Part model, mm, in its own coordinate system. Face numbers are marked on the shaded views. A direction names the side the tool comes from. Give positions to 0.01 mm unless a question says otherwise; leave off trailing zeros. Order: outer loops, then holes, each group sorted by start corner. A loop starts at its lowest first (then second) coordinate and runs counter-clockwise, first axis right, second up. Notation, with made-up numbers: M 66.25,75 L 81.25,75 A21 ccw 81.25,103 Z; hole C -36.5,29 d3. An arc over 180 degrees is marked long. One line per question, with ' | ' between items.
```python
from build123d import *

# Parameters (mm, degrees)
SKETCH1_W           = 200
SKETCH1_H           = 150
BOSS_EXTRUDE1_DEPTH = 150
SKETCH2_R           = 15
SKETCH2_R_2         = 13
BOSS_EXTRUDE2_DEPTH = 5
SKETCH3_R           = 13
SKETCH3_R_2         = 5
CUT_EXTRUDE1_DEPTH  = 70
CUT_EXTRUDE2_DEPTH  = 201
SKETCH5_R           = 15
SKETCH5_R_2         = 14
BOSS_EXTRUDE3_DEPTH = 10
SKETCH7_R           = 10
SKETCH7_R_2         = 9
SKETCH7_R_3         = 16
SKETCH7_R_4         = 15
BOSS_EXTRUDE4_DEPTH = 20
SKETCH10_W          = 70
SKETCH10_H          = 50
CUT_EXTRUDE5_DEPTH  = 151


with BuildPart() as part:
    # Sketch1 → Boss-Extrude1 (new body)
    with BuildSketch(Plane(origin=(0, 0, 0), x_dir=(1, 0, 0), z_dir=(0, 1, 0))):
        Rectangle(SKETCH1_W, SKETCH1_H)
    extrude(amount=BOSS_EXTRUDE1_DEPTH)

    # Sketch2 → Boss-Extrude2 (add)
    with BuildSketch(Plane(origin=(100, 0, 0), x_dir=(0, 0, -1), z_dir=(1, 0, 0))):
        with Locations((-10, 20)):
            Circle(SKETCH2_R)
        with Locations((-10, 20)):
            Circle(SKETCH2_R_2, mode=Mode.SUBTRACT)
    extrude(amount=BOSS_EXTRUDE2_DEPTH)

    # Sketch3 → Cut-Extrude1 (cut)
    with BuildSketch(Plane(origin=(100, 0, 0), x_dir=(0, 0, -1), z_dir=(1, 0, 0))):
        with Locations((-10, 20)):
            Circle(SKETCH3_R)
        with Locations((-37.5, 20)):
            Circle(SKETCH3_R_2)
        with Locations((17.5, 20)):
            Circle(SKETCH3_R_2)
        Polygon((75, 10), (20, 10), (20, 0), (20, -30), (75, -30), (75, 0), align=None)
    extrude(amount=-CUT_EXTRUDE1_DEPTH, mode=Mode.SUBTRACT)

    # Sketch4 → Cut-Extrude2 (cut, through all)
    with BuildSketch(Plane(origin=(100, 0, 0), x_dir=(0, 0, -1), z_dir=(1, 0, 0))):
        Polygon((-37.5, 150), (-75, 112.5), (-75, 150), align=None)
    extrude(amount=-CUT_EXTRUDE2_DEPTH, mode=Mode.SUBTRACT)

    # Sketch5 → Boss-Extrude3 (add)
    with BuildSketch(Plane(origin=(0, 93.75, 93.75), x_dir=(1, 0, 0), z_dir=(0, 0.707106781, 0.707106781))):
        with Locations((-50, 53.033008589)):
            Circle(SKETCH5_R)
        with Locations((-50, 53.033008589)):
            Circle(SKETCH5_R_2, mode=Mode.SUBTRACT)
    extrude(amount=BOSS_EXTRUDE3_DEPTH)

    # Sketch7 → Boss-Extrude4 (add)
    with BuildSketch(Plane(origin=(0, 150, 0), x_dir=(1, 0, 0), z_dir=(0, 1, 0))):
        Circle(SKETCH7_R)
        Circle(SKETCH7_R_2, mode=Mode.SUBTRACT)
        with Locations((-65.196037567, 0)):
            Circle(SKETCH7_R_3)
        with Locations((-65.196037567, 0)):
            Circle(SKETCH7_R_4, mode=Mode.SUBTRACT)
    extrude(amount=BOSS_EXTRUDE4_DEPTH)

    # Sketch10 → Cut-Extrude5 (cut, through all)
    with BuildSketch(Plane(origin=(0, 150, 0), x_dir=(1, 0, 0), z_dir=(0, 1, 0))):
        with Locations((65, 50)):
            Rectangle(SKETCH10_W, SKETCH10_H)
    extrude(amount=-CUT_EXTRUDE5_DEPTH, mode=Mode.SUBTRACT)


solid = part.part
```
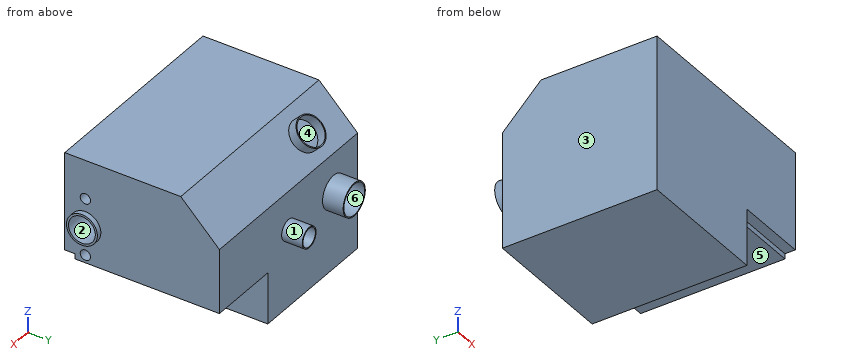
1. Probe L1, parallel to X at y = 159.25, z = 0; L2, parallel to Y at x = 45, z = -2; L3, parallel to X at y = 47.5, z = 51.5. List the from-to ranges inside material, lowest first. Write a range as from..to.
Worked out:
L1: x = -81.2..-80.2, -50.2..-49.2, -10..-9, 9..10 | L2: y = 0..15, 25..150 | L3: x = -100..100
2. Slice it at C-C on z = -35.5. Give the cut face in (x, y), then the cut area to 3 significant figures.
Worked out:
outline: M -100,0 L 30,0 L 30,150 L -100,150 Z | area: 19,500 mm2
3. Drop flat-ended pins along their axis: pin 1 (1.5 mm diameter, centred on x = 47.5, z = -23, fed in from -Y); pin 2 (9 mm diameter, centred on x = -70.5, z = 4.5, fed in from +Y); pin 3 (3 mm diameter, centred on x = 58.5, y = 5.5, fed in from -Z). Give the stop position or say it passes through.
Worked out:
pin 1: stops at y = 10 | pin 2: stops at y = 150 | pin 3: stops at z = -20
4. Tool access for the marked faces 4, 5 and 6: list every direction of +Z, -Z, +X, -X, +Y, -Y with a clear straight run to the whole face (end or side of a thin tool).
Worked out:
face 4: none | face 5: -Z, +X, +Y, -Y | face 6: +Y
5. Slice it at B-B on y = 39.5. Give the cut face in (x, z), then the cut area to 3 significant figures.
Worked out:
outline: M -100,-75 L 30,-75 L 30,-25 L 100,-25 L 100,75 L -100,75 Z | area: 26,500 mm2
6. Slice it at D-D on z = 0. Give the cut face in (x, y), then the cut area to 3 significant figures.
Worked out:
outline: M -100,0 L 100,0 L 100,8.82 L 105,8.82 L 105,11.69 L 30,11.69 L 30,28.31 L 105,28.31 L 105,31.18 L 100,31.18 L 100,150 L 10,150 L 10,170 L 9,170 L 9,150 L -9,150 L -9,170 L -10,170 L -10,150 L -49.2,150 L -49.2,170 L -50.2,170 L -50.2,150 L -80.2,150 L -80.2,170 L -81.2,170 L -81.2,150 L -100,150 Z | area: 28,900 mm2
7. Mould opens along Z. For the marked faces 1, 2 and 3 say: released by +Z, released by -Z, zero draft, split by the parting line, or undercut.
Worked out:
face 1: split by the parting line | face 2: undercut | face 3: zero draft
8. Slice it at A-A on x = -18.5. Give the cut face in (y, z), then the cut area to 3 significant figures.
Worked out:
outline: M 0,-75 L 150,-75 L 150,37.5 L 112.5,75 L 0,75 Z | area: 21,800 mm2
